from build123d import *

# Parameters (mm, degrees)
PAD_DEPTH       = 10
PAD001_DEPTH    = 20
SKETCH002_R     = 1.6
POCKET_DEPTH    = 17
POCKET001_DEPTH = 17
SKETCH004_R     = 1.956014
POCKET002_DEPTH = 57.501
SKETCH005_R     = 1.5
POCKET003_DEPTH = 30.001
CHAMFER_SIZE    = 6.9
CHAMFER001_SIZE = 6.9
FILLET_R        = 20.9
FILLET001_R     = 20.9


with BuildPart() as part:
    # Sketch → Pad (new body)
    with BuildSketch(Plane.XY):
        Polygon((30, 55.5), (30, 48.5), (10, 48.5), (10, 7), (30, 7), (30, 0), (0, 0), (0, 55.5), align=None)
    extrude(amount=PAD_DEPTH)

    # Sketch001 → Pad001 (new body)
    with BuildSketch(Plane(origin=(0, 0, 0), x_dir=(0, -1, 0), z_dir=(-1, 0, 0))):
        Polygon((0, 10), (0, 0), (11.18034, -10), (51.18034, -10), (51.18034, 20), (11.18034, 20), align=None)
    extrude(amount=-PAD001_DEPTH)

    # Sketch002 → Pocket (cut)
    with BuildSketch(Plane.XZ.offset(51.18034)):
        with Locations((10, 5)):
            Circle(SKETCH002_R)
    extrude(amount=-POCKET_DEPTH, mode=Mode.SUBTRACT)

    # Sketch003 → Pocket001 (cut)
    with BuildSketch(Plane.YZ.offset(20)):
        Polygon((-49.18034, 18), (-49.18034, -8), (-11.180357, -8), (-2, 0.211161), (-2, 9.788839), (-11.180357, 18), align=None)
    extrude(amount=-POCKET001_DEPTH, mode=Mode.SUBTRACT)

    # Sketch004 → Pocket002 (cut, through all)
    with BuildSketch(Plane.XZ.offset(2)):
        with Locations((16.870201, 4.538767)):
            Circle(SKETCH004_R)
    extrude(amount=-POCKET002_DEPTH, mode=Mode.SUBTRACT)

    # Sketch005 → Pocket003 (cut, through all)
    with BuildSketch(Plane(origin=(0, 0, -10), x_dir=(1, 0, 0), z_dir=(0, 0, -1))):
        with Locations((13.718381, 37.10752)):
            Circle(SKETCH005_R)
    extrude(amount=-POCKET003_DEPTH, mode=Mode.SUBTRACT)

    # Chamfer
    chamfer_edges = [part.edges().sort_by_distance(p)[0] for p in [
        (10, 0, 0),
    ]]
    chamfer(chamfer_edges, length=CHAMFER_SIZE)

    # Chamfer001
    chamfer001_edges = [part.edges().sort_by_distance(p)[0] for p in [
        (10, 0, 10),
    ]]
    chamfer(chamfer001_edges, length=CHAMFER001_SIZE)

    # Fillet
    fillet_edges = [part.edges().sort_by_distance(p)[0] for p in [
        (10, -11.18034, -10),
    ]]
    fillet(fillet_edges, radius=FILLET_R)

    # Fillet001
    fillet001_edges = [part.edges().sort_by_distance(p)[0] for p in [
        (10, -11.18034, 20),
    ]]
    fillet(fillet001_edges, radius=FILLET001_R)


solid = part.part
Geometry check sheet. Reference: the model listing, model coordinates, mm. A direction names the side the tool comes from. Round coordinates to 2 decimals unless told otherwise and drop trailing zeros. Loops run counter-clockwise (first coordinate to the right, second up) from the corner with the lowest first, then second, coordinate; pieces in that order, holes last. Notation, with made-up numbers: (6, -31) -> (51, -31) arc R24 ccw to (51, -14) -> close; hole circle Ø8 at (22, 32). An arc over 180 degrees is marked (long way). Answer as a JSON object with one key per item and string values. Group by question number.
Item 1: Cross-section at A-A, the plane x = 26.75. Record the cut outline in (y, z), plus the area to 3 significant figures.
Item 2: Cross-section at C-C, the plane z = -5.75. Record the cut outline in (x, y).
Item 3: Thickness scan on line 1 along Y through (x, z) = (13.5, 4); line 2 along Y through (x, z) = (26, 9); line 3 along Z through (x, y) = (6.5, -44.5). Record the ranges inside material, lowest first.
Item 4: Cross-section at B-B, the plane z = 8.5. Record the cut outline in (x, y), plus the area to 3 significant figures.
Item 5: Set-up check for faces 4 (the face through (25, 0, 5)), 5 (the face through (16.45, 2.44, 2.63)), 6 (the face through (12, -30, -8)), 7 (the face through (20, 48.5, 5)): record each of +Z, -Z, +X, -X, +Y, -Y from which the full face is reachable in a straight line by a thin tool's end or side.
Item 6: Release check for a two-part mould opening along Y. For faces 1 (the face through (11.62, -6.65, -3.95)), 2 (the face through (20, -26.3, 18.4)), 3 (the face through (12, -51.18, 5)) record: pulls with the +Y half, pulls with the -Y half, needs draft (parallel to the pull), parting line crosses it, or undercut.
Item 7: Depth check by flat-ended pin: pin 1 Ø15 at (x, y) = (12, 22) entering from +Z; pin 2 Ø2.5 at (x, y) = (13.72, -37.11) entering from -Z; pin 3 Ø1.5 at (y, z) = (9, 3) entering from +X; pin 4 Ø11 at (x, z) = (27, 6) entering from -Y. Enter the tip coordinate at first touch or a pass-through.
Determined:
{
 "1": {"outline": "(0, 0) -> (7, 0) -> (7, 10) -> (0, 10) -> close; (48.5, 0) -> (55.5, 0) -> (55.5, 10) -> (48.5, 10) -> close", "area": "140 mm²"},
 "2": {"outline": "(0, -51.18) -> (20, -51.18) -> (20, -49.18) -> (3, -49.18) -> (3, -8.66) -> (20, -8.66) -> (20, -6.53) -> (0, -6.53) -> close"},
 "3": {"line 1": "y = -51.18 to -49.18, -2 to 7, 48.5 to 55.5", "line 2": "y = 0 to 7, 48.5 to 55.5", "line 3": "z = -10 to -8, 18 to 20"},
 "4": {"outline": "(0, -51.18) -> (20, -51.18) -> (20, -49.18) -> (3, -49.18) -> (3, -2) -> (20, -2) -> (20, 0) -> (30, 0) -> (30, 7) -> (10, 7) -> (10, 48.5) -> (30, 48.5) -> (30, 55.5) -> (0, 55.5) -> close", "area": "1,060 mm²"},
 "5": {"face 4": "+Z, -Z, +X, -Y", "face 5": "+Y", "face 6": "+X", "face 7": "+Z, -Z, +X"},
 "6": {"face 1": "undercut", "face 2": "needs draft", "face 3": "pulls with the -Y half"},
 "7": {"pin 1": "stops at z = 10", "pin 2": "passes through", "pin 3": "stops at x = 10", "pin 4": "stops at y = 0"}
}
